Here's how the part is built. I have some questions about the finished solid (model axes, mm). A direction names the side the tool comes from. Give positions to 0.01 mm unless a question says otherwise; leave off trailing zeros. Loops run counter-clockwise (first coordinate to the right, second up) from the corner with the lowest first, then second, coordinate; pieces in that order, holes last.
Q1. Will these pins go through, and if not, where does the flat tip stop? P1, Ø13, axis at x = 3.5, y = 23.5, coming from the +Z side; P2, Ø3, axis at x = -12, y = 3, coming from the +Z side; P3, Ø10, axis at x = 8.5, z = -36, coming from the +Y side.
Q2. If we section it at C-C (x = 1.5): Please give me the cut outline in (y, z), plus the area to 3 significant figures.
Q3. If we section it at A-A (z = -21): Please give me the cut outline in (x, y), plus the area to 3 significant figures.
Q4. If we section it at D-D (y = 7.5): Please give me the cut outline in (x, z).
Q5. We'd pull the mould along X, two halves only. Please class faces 6 (the face through (-7, 23, -44)), 7 (the face through (0, 5, -36.5)), 8 (the face through (-3, 0, -38)), 9 (the face through (-0.378, 27.125, -46.703)): +X half, -X half, draft (parallel to the pull), parting line (faces both ways), or undercut.
Q6. I need wall thicknesses on line 1 (X direction, y = 9.5, z = -36); line 2 (Y direction, x = -5, z = -37); line 3 (Z direction, x = -19, y = 7). Which ranges of each line are inside material? Lowest first, please.
Q7. For faces 1 (the face through (0.521, 26.034, -38.043)), 2 (the face through (7, 23, -44)), 3 (the face through (35.7, 5, -12)), 4 (the face through (25.7, 5, -7)), 5 (the face through (-31, 5, 21.5)), which set-ups out of +Z, -Z, +X, -X, +Y, -Y let a thin tool reach every point of the face, with its end or its side?
Q8. If we section it at B-B (y = 30): Please give me the cut outline in (x, z).
from build123d import *

# Parameters (mm, degrees)
SKETCH2_W           = 71.4
SKETCH2_H           = 93
SKETCH2_W_2         = 51.4
SKETCH2_H_2         = 73
BOSS_EXTRUDE1_DEPTH = 10
SKETCH3_W           = 14
SKETCH3_H           = 26
SKETCH3_R           = 2.5
BOSS_EXTRUDE2_DEPTH = 5
SKETCH4_R           = 4
SKETCH4_R_2         = 2.5
BOSS_EXTRUDE3_DEPTH = 6.6
SKETCH5_W           = 51.4
SKETCH5_H           = 10
CUT_EXTRUDE1_DEPTH  = 65.130647899
SKETCH6_R           = 5.2
SKETCH6_R_2         = 4
BOSS_EXTRUDE4_DEPTH = 0.4
SKETCH7_W           = 71.4
SKETCH7_H           = 25
CUT_EXTRUDE2_DEPTH  = 65.130647899
BOSS_EXTRUDE5_START = 0.4
SKETCH8_R           = 2.9
SKETCH8_R_2         = 2.5
BOSS_EXTRUDE5_DEPTH = 0.4
FILLET1_START       = -46.5
FILLET1_DEPTH       = 5
FILLET1_2_DEPTH     = 5


with BuildPart() as part:
    # Sketch2 → Boss-Extrude1 (new body)
    with BuildSketch(Plane(origin=(0, 0, 0), x_dir=(1, 0, 0), z_dir=(0, 1, 0))):
        Rectangle(SKETCH2_W, SKETCH2_H)
        Rectangle(SKETCH2_W_2, SKETCH2_H_2, mode=Mode.SUBTRACT)
    extrude(amount=BOSS_EXTRUDE1_DEPTH)

    # Sketch3 → Boss-Extrude2 (add)
    with BuildSketch(Plane(origin=(0, 0, -46.5), x_dir=(-1, 0, 0), z_dir=(0, 0, -1))):
        with Locations((0, 23)):
            Rectangle(SKETCH3_W, SKETCH3_H)
        with Locations((0, 30)):
            Circle(SKETCH3_R, mode=Mode.SUBTRACT)
    extrude(amount=-BOSS_EXTRUDE2_DEPTH)

    # Sketch4 → Boss-Extrude3 (add)
    with BuildSketch(Plane.XY.offset(-41.5)):
        with Locations(Location((0, 30, 0), (0, 0, 180))):
            Circle(SKETCH4_R)
        with Locations(Location((0, 30, 0), (0, 0, 180))):
            Circle(SKETCH4_R_2, mode=Mode.SUBTRACT)
    extrude(amount=BOSS_EXTRUDE3_DEPTH)

    # Sketch5 → Cut-Extrude1 (cut, through all)
    with BuildSketch(Plane(origin=(0, 10, 0), x_dir=(1, 0, 0), z_dir=(0, 1, 0))):
        with Locations((0, -41.5)):
            Rectangle(SKETCH5_W, SKETCH5_H)
    extrude(amount=-CUT_EXTRUDE1_DEPTH, mode=Mode.SUBTRACT)

    # Sketch6 → Boss-Extrude4 (add)
    with BuildSketch(Plane.XY.offset(-41.5)):
        with Locations(Location((0, 30, 0), (0, 0, 180))):
            Circle(SKETCH6_R)
        with Locations((0, 30)):
            Circle(SKETCH6_R_2, mode=Mode.SUBTRACT)
    extrude(amount=BOSS_EXTRUDE4_DEPTH)

    # Sketch7 → Cut-Extrude2 (cut, through all)
    with BuildSketch(Plane(origin=(0, 10, 0), x_dir=(1, 0, 0), z_dir=(0, 1, 0))):
        with Locations((0, -34)):
            Rectangle(SKETCH7_W, SKETCH7_H)
    extrude(amount=-CUT_EXTRUDE2_DEPTH, mode=Mode.SUBTRACT)

    # Sketch8 → Boss-Extrude5 (add)
    with BuildSketch(Plane(origin=(0, 0, -46.5), x_dir=(-1, 0, 0), z_dir=(0, 0, -1)).offset(BOSS_EXTRUDE5_START)):
        with Locations(Location((0, 30, 0), (0, 0, 180))):
            Circle(SKETCH8_R)
        with Locations((0, 30)):
            Circle(SKETCH8_R_2, mode=Mode.SUBTRACT)
    extrude(amount=-BOSS_EXTRUDE5_DEPTH)

    # Fillet1: read off the stored shape, not the designer's step
    # Fillet1 outline → Fillet1 (cut)
    with BuildSketch(Plane.XY.offset(FILLET1_START)):
        with BuildLine():
            ThreePointArc((0, 36), (4.949747468, 33.949747468), (7, 29))
            Line((7, 29), (7, 36))
            Line((7, 36), (0, 36))
        make_face()
        with BuildLine():
            ThreePointArc((-7, 29), (-4.949747468, 33.949747468), (0, 36))
            Line((0, 36), (-7, 36))
            Line((-7, 36), (-7, 29))
        make_face()
    extrude(amount=FILLET1_DEPTH, mode=Mode.SUBTRACT)

    # Fillet1 2 outline → Fillet1 2 (add)
    with BuildSketch(Plane.XY.offset(FILLET1_START)):
        with BuildLine():
            ThreePointArc((14, 10), (9.050252532, 12.050252532), (7, 17))
            Line((7, 17), (7, 10))
            Line((7, 10), (14, 10))
        make_face()
        with BuildLine():
            Line((-14, 10), (-7, 10))
            Line((-7, 10), (-7, 17))
            ThreePointArc((-7, 17), (-9.050252532, 12.050252532), (-14, 10))
        make_face()
    extrude(amount=FILLET1_2_DEPTH)


solid = part.part
Check sheet entries:
1. P1: stops at z = -34.9
1. P2: stops at z = -36.5
1. P3: stops at y = 31.94
2. outline: (0, -46.5) - (27.52, -46.5) - (27.52, -46.9) - (28, -46.9) - (28, -34.9) - (26.29, -34.9) - (26.29, -41.1) - (25.02, -41.1) - (25.02, -41.5) - (10, -41.5) - (10, -36.5) - (0, -36.5) - close; (32, -46.9) - (32.48, -46.9) - (32.48, -46.5) - (35.84, -46.5) - (35.84, -41.5) - (34.98, -41.5) - (34.98, -41.1) - (33.71, -41.1) - (33.71, -34.9) - (32, -34.9) - close
2. area: 233 mm2
3. outline: (-35.7, 0) - (-25.7, 0) - (-25.7, 10) - (-35.7, 10) - close; (25.7, 0) - (35.7, 0) - (35.7, 10) - (25.7, 10) - close
3. area: 200 mm2
4. outline: (-35.7, -46.5) - (35.7, -46.5) - (35.7, 21.5) - (25.7, 21.5) - (25.7, -36.5) - (-25.7, -36.5) - (-25.7, 21.5) - (-35.7, 21.5) - close
5. face 6: -X half
5. face 7: undercut
5. face 8: draft
5. face 9: parting line
6. line 1: x = -35.7 to -25.7, 25.7 to 35.7
6. line 2: y = 0 to 10
6. line 3: z = -46.5 to -36.5
7. face 1: +Z
7. face 2: +Z, -Z, +X, +Y
7. face 3: +Z, -Z, +X, +Y, -Y
7. face 4: +Z, +Y, -Y
7. face 5: +Z, +X, -X, +Y, -Y
8. outline: (-6.93, -46.5) - (-2.9, -46.5) - (-2.9, -46.9) - (-2.5, -46.9) - (-2.5, -34.9) - (-4, -34.9) - (-4, -41.1) - (-5.2, -41.1) - (-5.2, -41.5) - (-6.93, -41.5) - close; (2.5, -46.9) - (2.9, -46.9) - (2.9, -46.5) - (6.93, -46.5) - (6.93, -41.5) - (5.2, -41.5) - (5.2, -41.1) - (4, -41.1) - (4, -34.9) - (2.5, -34.9) - close
